The listing builds one solid part. Answer for the finished solid, in the listing's coordinates (mm). Give positions to 0.01 mm unless a question says otherwise; leave off trailing zeros. Write each loop counter-clockwise with the first axis right and the second up, starting at its lowest first coordinate (ties: lowest second). Pieces come first, ordered by that corner, then holes. Notation, with made-up numbers: (23, -11.5) - (63, -11.5) arc R24 ccw to (63, 7.5) - close; hole circle Ø1 at (-30, 1). An arc over 180 degrees is marked (long way). Write each question's results on one line, items separated by ' | '. Start each with the question number.
Q1. Find the intervals of material crossed by probe 1 along Y at (x, z) = (336, 2.3); probe 2 along Y at (x, z) = (336.55, 1.8) (3 decimals); probe 3 along X at (y, z) = (279, 1.6), in increasing order.
Q2. Section A-A (y = 276.5) is taken. Determine the outline of the cut face in (x, z) (3 decimals), plus the area to 3 significant figures.
Q3. Section B-B (z = 1.85) is taken. State how many separate pieces and enclosed holes the cut face has, plus the area to 3 significant figures.
Q4. Flat-ended cylindrical pins translate along their axes: pin 1 Ø6.5 at (x, y) = (336.55, 75.565) entering from -Z; pin 2 Ø1 at (y, z) = (440, 1.5) entering from -X (3 decimals); pin 3 Ø1.6 at (x, z) = (233, 1) entering from -Y. Find the tip coordinate at first contact, or state that the pin passes through.
Q5. Section C-C (x = 204.5) is taken. Determine the outline of the cut face in (y, z) (3 decimals), plus the area to 3 significant figures.
```python
from build123d import *

# Parameters (mm, degrees)
SKETCH1_W           = 539.75
SKETCH1_H           = 508
BOSS_EXTRUDE1_DEPTH = 3.175
SKETCH2_R           = 2.54
SKETCH2_R_2         = 3.175
SKETCH2_W           = 177.8
SKETCH2_H           = 292.1
CUT_EXTRUDE1_DEPTH  = 44.45
SKETCH3_W           = 34.925
SKETCH3_H           = 127
CUT_EXTRUDE2_DEPTH  = 742.218013222
SKETCH4_R           = 1.8034
CUT_EXTRUDE3_DEPTH  = 742.218013222
SKETCH5_R           = 2.54
CUT_EXTRUDE4_DEPTH  = 742.218013222
SKETCH6_R           = 2.54
CUT_EXTRUDE5_DEPTH  = 742.218013222


with BuildPart() as part:
    # Sketch1 → Boss-Extrude1 (new body)
    with BuildSketch(Plane.XY):
        with Locations((269.875, 254)):
            Rectangle(SKETCH1_W, SKETCH1_H)
    extrude(amount=BOSS_EXTRUDE1_DEPTH)

    # Sketch2 → Cut-Extrude1 (cut)
    with BuildSketch(Plane(origin=(0, 0, 0), x_dir=(-1, 0, 0), z_dir=(0, 0, -1))):
        with Locations((-336.55, 45.085)):
            Circle(SKETCH2_R)
        with Locations((-146.05, 45.085)):
            Circle(SKETCH2_R)
        with Locations((-15.24, 365.76)):
            Circle(SKETCH2_R_2)
        with Locations((-241.3, 146.05)):
            Rectangle(SKETCH2_W, SKETCH2_H)
    extrude(amount=-CUT_EXTRUDE1_DEPTH, mode=Mode.SUBTRACT)

    # Sketch3 → Cut-Extrude2 (cut, through all)
    with BuildSketch(Plane(origin=(0, 0, 0), x_dir=(-1, 0, 0), z_dir=(0, 0, -1))):
        with Locations((-17.4625, 444.5)):
            Rectangle(SKETCH3_W, SKETCH3_H)
    extrude(amount=-CUT_EXTRUDE2_DEPTH, mode=Mode.SUBTRACT)

    # Sketch4 → Cut-Extrude3 (cut, through all)
    with BuildSketch(Plane(origin=(0, 0, 0), x_dir=(-1, 0, 0), z_dir=(0, 0, -1))):
        with Locations((-311.1754, 297.6372)):
            Circle(SKETCH4_R)
        with Locations((-295.3004, 297.6372)):
            Circle(SKETCH4_R)
        with Locations((-187.3504, 297.6372)):
            Circle(SKETCH4_R)
        with Locations((-171.4754, 297.6372)):
            Circle(SKETCH4_R)
    extrude(amount=-CUT_EXTRUDE3_DEPTH, mode=Mode.SUBTRACT)

    # Sketch5 → Cut-Extrude4 (cut, through all)
    with BuildSketch(Plane.XY.offset(3.175)):
        with Locations((146.05, 75.565)):
            Circle(SKETCH5_R)
    extrude(amount=-CUT_EXTRUDE4_DEPTH, mode=Mode.SUBTRACT)

    # Sketch6 → Cut-Extrude5 (cut, through all)
    with BuildSketch(Plane.XY.offset(3.175)):
        with Locations((336.55, 75.565)):
            Circle(SKETCH6_R)
    extrude(amount=-CUT_EXTRUDE5_DEPTH, mode=Mode.SUBTRACT)


solid = part.part
```
Answers below:
1) probe 1: y = 0 to 42.61, 47.56 to 73.09, 78.04 to 508 | probe 2: y = 0 to 42.545, 47.625 to 73.025, 78.105 to 508 | probe 3: x = 0 to 152.4, 330.2 to 539.75
2) outline: (0, 0) - (152.4, 0) - (152.4, 3.175) - (0, 3.175) - close; (330.2, 0) - (539.75, 0) - (539.75, 3.175) - (330.2, 3.175) - close | area: 1,150 mm2
3) separate pieces: 1 | enclosed holes: 9 | area: 218,000 mm2
4) pin 1: stops at z = 0 | pin 2: stops at x = 34.925 | pin 3: stops at y = 292.1
5) outline: (292.1, 0) - (508, 0) - (508, 3.175) - (292.1, 3.175) - close | area: 685 mm2
